Check sheet for the modelled part. Datum: model origin and axes. Units: mm. A direction names the side the tool comes from. Coordinates: 2 decimals unless noted, no trailing zeros. Order: outer loops, then holes, each group sorted by start corner. A loop starts at its lowest first (then second) coordinate and runs counter-clockwise, first axis right, second up.
from build123d import *

# Parameters (mm, degrees)
SKETCH1_W           = 863.6
SKETCH1_H           = 863.6
SKETCH1_W_2         = 711.2
SKETCH1_H_2         = 711.2
EXTRUDE_THIN1_DEPTH = 76.2
FILLET1_R           = 30


with BuildPart() as part:
    # Sketch1 → Extrude-Thin1 (new body)
    with BuildSketch(Plane(origin=(0, 0, 0), x_dir=(1, 0, 0), z_dir=(0, 1, 0))):
        with Locations((-355.6, -355.6)):
            Rectangle(SKETCH1_W, SKETCH1_H)
        with Locations((-355.6, -355.6)):
            Rectangle(SKETCH1_W_2, SKETCH1_H_2, mode=Mode.SUBTRACT)
    extrude(amount=EXTRUDE_THIN1_DEPTH)

    # Fillet1
    fillet1_edges = [part.edges().sort_by_distance(p)[0] for p in [
        (-787.4, 76.2, 355.6),
        (-355.6, 76.2, 787.4),
        (-355.6, 0, 787.4),
        (-787.4, 0, 355.6),
        (-355.6, 0, -76.2),
        (76.2, 0, 355.6),
        (76.2, 76.2, 355.6),
        (76.2, 38.1, 787.4),
        (-787.4, 38.1, 787.4),
        (-787.4, 38.1, -76.2),
        (76.2, 38.1, -76.2),
        (-355.6, 76.2, -76.2),
    ]]
    fillet(fillet1_edges, radius=FILLET1_R)


solid = part.part
(1) Release check for a two-part mould opening along Z. For faces 3 (the cylindrical face through (-349.975, 67.179, -67.645)), 4 (the cylindrical face through (-778.845, 38.213, 778.379)), 5 (the cylindrical face through (-778.845, 9.021, 349.975)), 6 (the flat face through (-711.2, 38, 361)) record: +Z half, -Z half, draft (parallel to the pull), parting line (faces both ways), or undercut.
Filled in:
face 3: -Z half
face 4: +Z half
face 5: draft
face 6: undercut
(2) Thickness scan on probe 1 along Z at (x, y) = (-698.5, 43.5); probe 2 along X at (y, z) = (34, 472.5); probe 3 along X at (y, z) = (48.5, 112.5). Record the ranges inside material, lowest first.
Filled in:
probe 1: z = -76.2 to 0, 711.2 to 787.4
probe 2: x = -787.4 to -711.2, 0 to 76.2
probe 3: x = -787.31 to -711.2, 0 to 76.11
(3) Tool access check on faces 1 (the cylindrical face through (67.645, 9.021, 349.975)), 2 (the flat face through (-361, 38, 711.2)). Record the directions out of +Z, -Z, +X, -X, +Y, -Y that give a thin tool (end or side, any length) a straight path to the whole face; none if there is none.
Filled in:
face 1: +Z, -Z, +X, -Y
face 2: +Y, -Y
(4) Cross-section at D-D (y = 64). Enter the section's corners in (x, z).
Filled in:
outline: (-781.55, -46.2) arc R24.15 ccw to (-757.4, -70.35) - (46.2, -70.35) arc R24.15 ccw to (70.35, -46.2) - (70.35, 757.4) arc R24.15 ccw to (46.2, 781.55) - (-757.4, 781.55) arc R24.15 ccw to (-781.55, 757.4) - close; hole (-711.2, 0) - (0, 0) - (0, 711.2) - (-711.2, 711.2) - close
(5) Cross-section at A-A (x = -516). Enter the section's corners in (y, z).
Filled in:
outline: (0, -46.2) arc R30 ccw to (30, -76.2) - (46.2, -76.2) arc R30 ccw to (76.2, -46.2) - (76.2, 0) - (0, 0) - close; (0, 711.2) - (76.2, 711.2) - (76.2, 757.4) arc R30 ccw to (46.2, 787.4) - (30, 787.4) arc R30 ccw to (0, 757.4) - close
(6) Cross-section at B-B (z = 466). Enter the section's corners in (x, y).
Filled in:
outline: (-787.4, 30) arc R30 ccw to (-757.4, 0) - (-711.2, 0) - (-711.2, 76.2) - (-757.4, 76.2) arc R30 ccw to (-787.4, 46.2) - close; (0, 0) - (46.2, 0) arc R30 ccw to (76.2, 30) - (76.2, 46.2) arc R30 ccw to (46.2, 76.2) - (0, 76.2) - close
(7) Go/stop test with flat-tipped pins: P1, Ø1, axis at y = 29, z = 72.5, coming from the -X side; P2, Ø12, axis at x = -353, y = 15.5, coming from the -Z side; P3, Ø2, axis at y = 61.5, z = 110.5, coming from the +X side. Record where each tip stops, or that it passes through.
Filled in:
P1: stops at x = -787.4
P2: stops at z = -74.97
P3: stops at x = 72.57
(8) Cross-section at C-C (y = 11.5). Enter the section's corners in (x, z), and give its area (3 significant figures).
Filled in:
outline: (-781.02, -46.2) arc R23.62 ccw to (-757.4, -69.82) - (46.2, -69.82) arc R23.62 ccw to (69.82, -46.2) - (69.82, 757.4) arc R23.62 ccw to (46.2, 781.02) - (-757.4, 781.02) arc R23.62 ccw to (-781.02, 757.4) - close; hole (-711.2, 0) - (0, 0) - (0, 711.2) - (-711.2, 711.2) - close
area: 218,000 mm2
